Answer from the drawing. Dimensions are ordinates in mm from the lowest x, y and z of the part. A direction names the side the tool comes from. Round coordinates to 2 decimals unless told otherwise and drop trailing zeros. Write each loop counter-clockwise with the first axis right and the second up, starting at its lowest first coordinate (ties: lowest second). Pieces come first, ordered by that corner, then holes. Notation, with made-up numbers: (-5.5, 1) - (31.5, 1) arc R34 cw to (31.5, 38) - close; hole circle Ø8 at (71, 60). An arc over 180 degrees is marked (long way). Use a Markdown table: item, result. Add a question column.
1) A cutting plane is placed at A-A (x = 7). Give the vertices of the cut face in (y, z).
2) A cutting plane is placed at B-B (z = 6.5). Give the vertices of the cut face in (x, y), then the cut area to 3 significant figures.
3) A tool of negligible diameter and unlimited length cuts with its end or side. For the marked faces 5, 6 and 7, from which of +Z, -Z, +X, -X, +Y, -Y can it reach the whole face along a straight path? Write none if from no direction.
4) A cutting plane is placed at D-D (x = 10.5). Give the vertices of the cut face in (y, z).
5) Find the intervals of material crossed by probe 1 along X at (y, z) = (2.2, 6.5); probe 2 along Z at (x, y) = (3.5, 1.35); probe 3 along Z at (x, y) = (7.5, 1.5), in increasing order. Write a range as from..to.
6) A cutting plane is placed at C-C (y = 0.75). Give the vertices of the cut face in (x, z).
7) Determine the mould class of the marked faces 1, 2, 3 and 4 for opening direction Z: +Z half, -Z half, draft (parallel to the pull), parting line (faces both ways), or undercut.
8) Each of these flat-tipped pins is pushed along its axis until it touches: P1, Ø1.5, axis at y = 2, z = 1.5, coming from the +X side; P2, Ø0.9, axis at x = 1.5, y = 1, coming from the -Z side; P3, Ø1.8, axis at x = 7, z = 6.5, coming from the +Y side; P4, Ø0.9, axis at y = 1.5, z = 1.5, coming from the -X side. Where does it stop, or does it pass through?
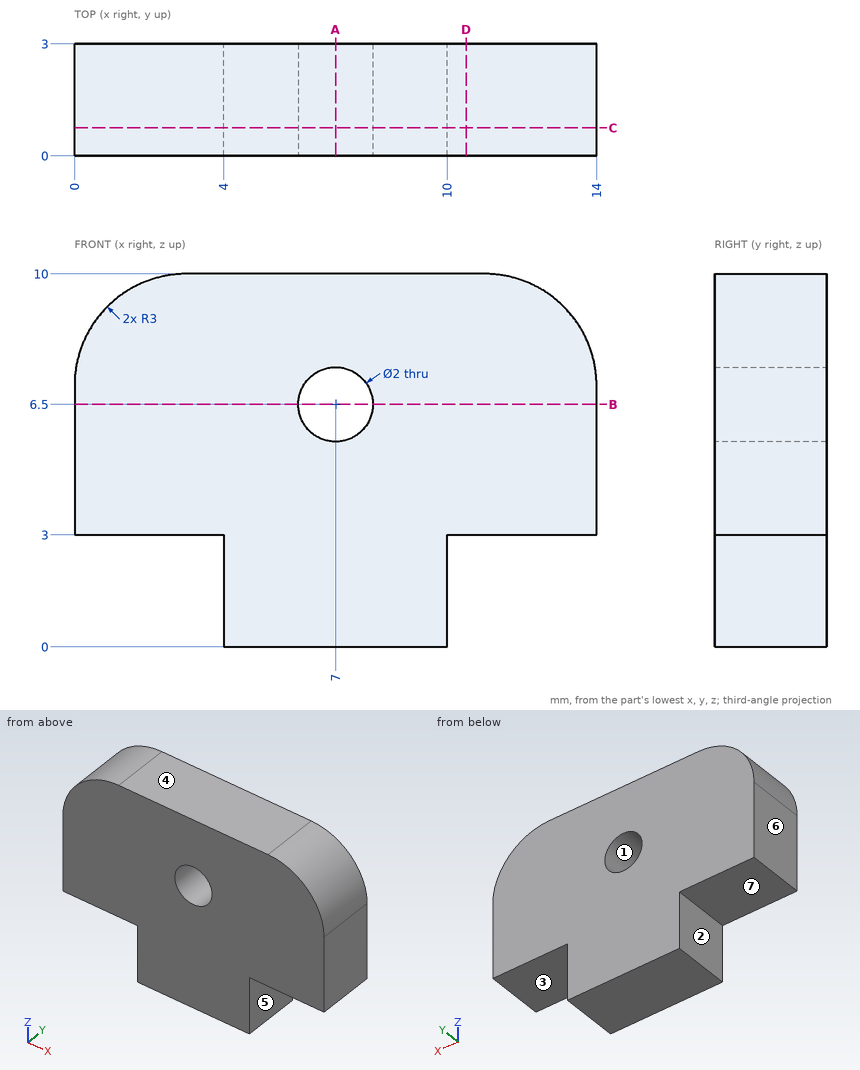
Entries:
| question | item | result |
|---|---|---|
| 1 | outline | (0, 0) - (3, 0) - (3, 5.5) - (0, 5.5) - close; (0, 7.5) - (3, 7.5) - (3, 10) - (0, 10) - close |
| 2 | outline | (0, 0) - (6, 0) - (6, 3) - (0, 3) - close; (8, 0) - (14, 0) - (14, 3) - (8, 3) - close |
| 2 | area | 36.0 mm² |
| 3 | face 5 | -Z, +X, +Y, -Y |
| 3 | face 6 | +Z, -Z, -X, +Y, -Y |
| 3 | face 7 | -Z, -X, +Y, -Y |
| 4 | outline | (0, 3) - (3, 3) - (3, 10) - (0, 10) - close |
| 5 | probe 1 | x = 0..6, 8..14 |
| 5 | probe 2 | z = 3..10 |
| 5 | probe 3 | z = 0..5.63, 7.37..10 |
| 6 | outline | (0, 3) - (4, 3) - (4, 0) - (10, 0) - (10, 3) - (14, 3) - (14, 7) arc R3 ccw to (11, 10) - (3, 10) arc R3 ccw to (0, 7) - close; hole circle Ø2 at (7, 6.5) |
| 7 | face 1 | undercut |
| 7 | face 2 | draft |
| 7 | face 3 | -Z half |
| 7 | face 4 | +Z half |
| 8 | P1 | stops at x = 10 |
| 8 | P2 | stops at z = 3 |
| 8 | P3 | passes through |
| 8 | P4 | stops at x = 4 |
